Input: part model. Units: mm. Frame: model coordinates. Face numbers are marked on the shaded views. A direction names the side the tool comes from. Round coordinates to 2 decimals unless told otherwise and drop trailing zeros. Order: outer loops, then holes, each group sorted by start corner. A loop starts at its lowest first (then second) coordinate and runs counter-clockwise, first axis right, second up. Notation, with made-up numbers: M -0.75,22 L 10.25,22 A14 cw 10.25,27 Z; hole C 14,6.25 d4. An arc over 180 degrees is marked long. One line per question, with ' | ' between items.
```python
from build123d import *

# Parameters (mm, degrees)
SKETCH1_W           = 15
SKETCH1_H           = 10
SKETCH1_R           = 1.7
SKETCH1_W_2         = 10
SKETCH1_H_2         = 15
BOSS_EXTRUDE1_DEPTH = 60
SKETCH2_W           = 5.8
SKETCH2_H           = 2.6
CUT_EXTRUDE1_DEPTH  = 9
SKETCH3_W           = 5.8
SKETCH3_H           = 2.6
CUT_EXTRUDE2_DEPTH  = 9
FILLET1_R           = 1
FILLET3_R           = 3
FILLET4_R           = 1


with BuildPart() as part:
    # Sketch1 → Boss-Extrude1 (new body)
    # profile 1 of 3: a face of its own
    with BuildSketch(Plane(origin=(0, 0, 0), x_dir=(1, 0, 0), z_dir=(0, 1, 0))):
        with Locations((-7.5, -5)):
            Rectangle(SKETCH1_W, SKETCH1_H)
        with Locations(Location((-10, -5, 0), (0, 0, 270))):
            Circle(SKETCH1_R, mode=Mode.SUBTRACT)
    # profile 2 of 3: a face of its own
    with BuildSketch(Plane(origin=(0, 0, 0), x_dir=(1, 0, 0), z_dir=(0, 1, 0))):
        with BuildLine():
            ThreePointArc((10, 0), (7.071067812, -7.071067812), (0, -10))
            Line((0, -10), (0, 0))
            Line((0, 0), (10, 0))
        make_face()
    # profile 3 of 3: a face of its own
    with BuildSketch(Plane(origin=(0, 0, 0), x_dir=(1, 0, 0), z_dir=(0, 1, 0))):
        with Locations((5, 7.5)):
            Rectangle(SKETCH1_W_2, SKETCH1_H_2)
        with Locations(Location((5, 10, 0), (0, 0, 270))):
            Circle(SKETCH1_R, mode=Mode.SUBTRACT)
    extrude(amount=BOSS_EXTRUDE1_DEPTH)

    # Sketch2 → Cut-Extrude1 (cut)
    with BuildSketch(Plane.ZY):
        with Locations((-10, 55)):
            Rectangle(SKETCH2_W, SKETCH2_H)
        with Locations((-10, 5)):
            Rectangle(SKETCH2_W, SKETCH2_H)
    extrude(amount=-CUT_EXTRUDE1_DEPTH, mode=Mode.SUBTRACT)

    # Sketch3 → Cut-Extrude2 (cut)
    with BuildSketch(Plane(origin=(0, 0, 0), x_dir=(-1, 0, 0), z_dir=(0, 0, -1))):
        with Locations((10, 55)):
            Rectangle(SKETCH3_W, SKETCH3_H)
        with Locations((10, 5)):
            Rectangle(SKETCH3_W, SKETCH3_H)
    extrude(amount=-CUT_EXTRUDE2_DEPTH, mode=Mode.SUBTRACT)

    # Fillet1
    fillet1_edges = [part.edges().sort_by_distance(p)[0] for p in [
        (0, 30, -15),
        (10, 30, -15),
        (-15, 30, 10),
        (-15, 30, 0),
    ]]
    fillet(fillet1_edges, radius=FILLET1_R)

    # Fillet3
    fillet3_edges = [part.edges().sort_by_distance(p)[0] for p in [
        (0, 30, 0),
    ]]
    fillet(fillet3_edges, radius=FILLET3_R)

    # Fillet4
    fillet4_edges = [part.edges().sort_by_distance(p)[0] for p in [
        (10, 0, -7),
        (5, 0, -15),
        (-15, 0, 5),
        (9.707106781, 0, -14.707106781),
        (0.292893219, 0, -14.707106781),
        (-14.707106781, 0, 0.292893219),
        (7.071067812, 0, 7.071067812),
        (-14.707106781, 0, 9.707106781),
        (-15, 60, 5),
        (5, 60, -15),
        (9.707106781, 60, -14.707106781),
        (-7, 0, 10),
        (0.292893219, 60, -14.707106781),
        (-14.707106781, 60, 0.292893219),
        (-14.707106781, 60, 9.707106781),
        (-8.5, 0, 0),
        (-8.5, 60, 0),
        (0, 60, -8.5),
        (0, 0, -8.5),
        (-0.878679656, 0, -0.878679656),
        (-0.878679656, 60, -0.878679656),
        (-7, 60, 10),
        (7.071067812, 60, 7.071067812),
        (10, 60, -7),
    ]]
    fillet(fillet4_edges, radius=FILLET4_R)


solid = part.part
```
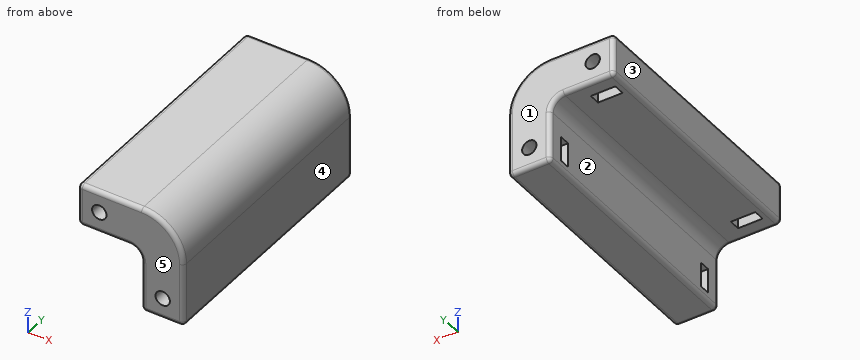
Item 1: Section query A-A, the plane x = -10. Return loops of the section in (y, z), plus the area to 3 significant figures.
Report:
outline: M 0,1 A1 ccw 1,0 L 3.7,0 L 3.7,3.3 L 0,3.3 Z; M 0,6.7 L 3.7,6.7 L 3.7,9 L 6.3,9 L 6.3,6.7 L 53.7,6.7 L 53.7,9 L 56.3,9 L 56.3,6.7 L 60,6.7 L 60,9 A1 ccw 59,10 L 1,10 A1 ccw 0,9 Z; M 6.3,0 L 53.7,0 L 53.7,3.3 L 6.3,3.3 Z; M 56.3,0 L 59,0 A1 ccw 60,1 L 60,3.3 L 56.3,3.3 Z | area: 366 mm²
Item 2: Section query C-C, the plane y = 29. Return loops of the section in (x, z), plus the area to 3 significant figures.
Report:
outline: M -15,1 A1 ccw -14,0 L -3,0 A3 cw 0,-3 L 0,-14 A1 ccw 1,-15 L 9,-15 A1 ccw 10,-14 L 10,0 A10 ccw 0,10 L -14,10 A1 ccw -15,9 Z; hole C -10,5 d3.4; hole C 5,-10 d3.4 | area: 361 mm²
Item 3: Mould query, pull axis X, two halves, no side actions, for the marked faces 3, 4 and 5. Classes: +X half, -X half, draft (parallel to the pull), parting line (faces both ways), or undercut.
Report:
face 3: -X half | face 4: +X half | face 5: draft
Item 4: Section query B-B, the plane z = -10. Return loops of the section in (x, y).
Report:
outline: M 0,1 A1 ccw 1,0 L 3.3,0 L 3.3,3.7 L 0,3.7 Z; M 0,6.3 L 3.3,6.3 L 3.3,53.7 L 0,53.7 Z; M 0,56.3 L 3.3,56.3 L 3.3,60 L 1,60 A1 ccw 0,59 Z; M 6.7,0 L 9,0 A1 ccw 10,1 L 10,59 A1 ccw 9,60 L 6.7,60 L 6.7,56.3 L 9,56.3 L 9,53.7 L 6.7,53.7 L 6.7,6.3 L 9,6.3 L 9,3.7 L 6.7,3.7 Z
Item 5: Line query: line 1 along Y through (x, z) = (5.25, -8); line 2 along Z through (x, y) = (-10, 27). Output: solid intervals per line, ascending. Write a range as from..to.
Report:
line 1: 0..3.7, 6.3..53.7, 56.3..60 | line 2: 0..3.3, 6.7..10
Item 6: First-contact query: pin 1 (3 mm diameter, centred on x = -11.5, y = 55, fed in from -Z); pin 2 (1 mm diameter, centred on y = 12.5, z = 2.5, fed in from +X); pin 3 (0.8 mm diameter, centred on y = 54.5, z = -9, fed in from -X). Flat tips, straight axial feed; report the tip coordinate or a pass-through.
Report:
pin 1: z = 0 | pin 2: x = 9.8 | pin 3: x = 9
Item 7: Section query D-D, the plane z = 8.25. Give the number of separate pieces and of enclosed holes in the cut face, plus the area to 3 significant figures.
Report:
separate pieces: 1 | enclosed holes: 2 | area: 1,210 mm²
Item 8: Access query for the marked faces 1 and 2. Directions: +Z, -Z, +X, -X, +Y, -Y. A direction counts if a zero-diameter tool reaches every point of the face in a straight line with its end or side. Return the directions, or none.
Report:
face 1: +Z, -Z, +X, -X, +Y | face 2: -Z, -X, +Y, -Y
